```python
from build123d import *

# Parameters (mm, degrees)
SKETCH_W        = 57
SKETCH_H        = 42
PAD_DEPTH       = 2
SKETCH001_W     = 57
SKETCH001_H     = 42
SKETCH001_W_2   = 53
SKETCH001_H_2   = 38
PAD001_DEPTH    = 2
SKETCH002_R     = 4
PAD002_DEPTH    = 12
SKETCH003_R     = 3.25
POCKET_DEPTH    = 14
SKETCH004_R     = 1.5
PAD003_DEPTH    = 2
POCKET001_DEPTH = 3
SKETCH006_W     = 26.076656
SKETCH006_H     = 2.5
POCKET002_DEPTH = 1
POCKET003_DEPTH = 1
PAD004_DEPTH    = 1
PAD005_DEPTH    = 17
PAD006_DEPTH    = 1
SKETCH011_W     = 42
SKETCH011_H     = 14
PAD007_DEPTH    = 1
SKETCH012_R     = 3.5
POCKET004_DEPTH = 2
SKETCH013_W     = 18
SKETCH013_H     = 38
PAD008_DEPTH    = 1
SKETCH014_W     = 0.782134
SKETCH014_H     = 1
PAD009_DEPTH    = 2
POCKET005_DEPTH = 15
POCKET006_DEPTH = 15
POCKET007_DEPTH = 3
POCKET008_DEPTH = 3
POCKET009_DEPTH = 80
POCKET010_DEPTH = 80
POCKET011_DEPTH = 42
POCKET012_DEPTH = 42


with BuildPart() as part:
    # Sketch → Pad (new body)
    with BuildSketch(Plane.XY):
        Rectangle(SKETCH_W, SKETCH_H)
    extrude(amount=PAD_DEPTH)

    # Sketch001 (on Face6 of Pad) → Pad001 (join)
    with BuildSketch(Plane.XY.offset(2)):
        Rectangle(SKETCH001_W, SKETCH001_H)
        Rectangle(SKETCH001_W_2, SKETCH001_H_2, mode=Mode.SUBTRACT)
    extrude(amount=PAD001_DEPTH)

    # Sketch002 (on Face4 of Pad001) → Pad002 (join)
    with BuildSketch(Plane(origin=(0, 0, 0), x_dir=(1, 0, 0), z_dir=(0, 0, -1))):
        with Locations((-12, 0)):
            Circle(SKETCH002_R)
    pad002 = extrude(amount=PAD002_DEPTH)

    # Sketch003 (on Face12 of Pad002) → Pocket (cut)
    with BuildSketch(Plane(origin=(0, 0, -12), x_dir=(1, 0, 0), z_dir=(0, 0, -1))):
        with Locations((-12, 0)):
            Circle(SKETCH003_R)
    pocket = extrude(amount=-POCKET_DEPTH, mode=Mode.SUBTRACT)

    # Mirrored: Pad002 across Sketch002 V_Axis
    add(pad002.mirror(Plane(origin=(0, 0, 0), x_dir=(0, 0, -1), z_dir=(1, 0, 0))))

    # Mirrored001: Pocket across Sketch003 V_Axis
    add(pocket.mirror(Plane(origin=(0, 0, -12), x_dir=(0, 0, -1), z_dir=(1, 0, 0))), mode=Mode.SUBTRACT)

    # Sketch004 (on Face21 of Mirrored001) → Pad003 (join)
    with BuildSketch(Plane.XY.offset(2)):
        with Locations((0, 12.5)):
            Circle(SKETCH004_R)
    pad003 = extrude(amount=PAD003_DEPTH)

    # Mirrored002: Pad003 across Sketch004 H_Axis
    add(pad003.mirror(Plane(origin=(0, 0, 2), x_dir=(0, 0, 1), z_dir=(0, 1, 0))))

    # Sketch005 (on Face21 of Mirrored002) → Pocket001 (cut)
    with BuildSketch(Plane.XY.offset(4)):
        with BuildLine():
            ThreePointArc((14.048565, -2.52307), (15.249949, -0.018175), (14.076656, 2.5))
            Line((14.076656, 2.5), (28.5, 2.5))
            Line((28.5, 2.5), (28.5, -21))
            Line((28.5, -21), (14.048565, -2.52307))
        make_face()
    extrude(amount=-POCKET001_DEPTH, mode=Mode.SUBTRACT)

    # Sketch006 (on Face17 of Pocket001) → Pocket002 (cut)
    with BuildSketch(Plane.XY.offset(2)):
        with Locations((1.038328, 1.25)):
            Rectangle(SKETCH006_W, SKETCH006_H)
    extrude(amount=-POCKET002_DEPTH, mode=Mode.SUBTRACT)

    # Sketch007 (on Face13 of Pocket002) → Pocket003 (cut)
    with BuildSketch(Plane.XY.offset(4)):
        Polygon((28.5, 21), (28.5, 20), (-27.5, 20), (-27.5, -20), (28.5, -20), (28.5, -21), (-28.5, -21), (-28.5, 21), align=None)
    extrude(amount=-POCKET003_DEPTH, mode=Mode.SUBTRACT)

    # Sketch008 (on Face3 of Pocket003) → Pad004 (join)
    with BuildSketch(Plane.YZ.offset(28.5)):
        Polygon((-19, 1), (-19, 15), (-20, 15), (-20, 4), (-20, 3), (-21, 3), (-21, 0), (21, 0), (21, 3), (20, 3), (20, 15), (19, 15), (19, 1), align=None)
    extrude(amount=PAD004_DEPTH)

    # Sketch009 (on Face10 of Pad004) → Pad005 (join)
    with BuildSketch(Plane.YZ.offset(29.5)):
        Polygon((-19, 15), (-20, 15), (-20, 14), (-21, 14), (-21, 0), (21, 0), (21, 14), (20, 14), (20, 15), (19, 15), (19, 1), (-19, 1), align=None)
    extrude(amount=PAD005_DEPTH)

    # Sketch010 (on Face20 of Pad005) → Pad006 (join)
    with BuildSketch(Plane.YZ.offset(46.5)):
        Polygon((-20, 15), (20, 15), (20, 14), (21, 14), (21, 0), (-21, 0), (-21, 14), (-20, 14), align=None)
    extrude(amount=PAD006_DEPTH)

    # Sketch011 (on Face34 of Pad006) → Pad007 (join)
    with BuildSketch(Plane.YZ.offset(47.5)):
        with Locations((0, 7)):
            Rectangle(SKETCH011_W, SKETCH011_H)
    extrude(amount=PAD007_DEPTH)

    # Sketch012 (on Face51 of Pad007) → Pocket004 (cut)
    with BuildSketch(Plane.YZ.offset(48.5)):
        with Locations((0, 8.5)):
            Circle(SKETCH012_R)
    extrude(amount=-POCKET004_DEPTH, mode=Mode.SUBTRACT)

    # Sketch013 (on Face77 of Pocket004) → Pad008 (join)
    with BuildSketch(Plane.XY.offset(1)):
        with Locations((37.5, 0)):
            Rectangle(SKETCH013_W, SKETCH013_H)
    extrude(amount=PAD008_DEPTH)

    # Sketch014 (on Face40 of Pad008) → Pad009 (join)
    with BuildSketch(Plane.XY.offset(1)):
        with Locations((28.108933, -20.5)):
            Rectangle(SKETCH014_W, SKETCH014_H)
    extrude(amount=PAD009_DEPTH)

    # Sketch015 (on Face50 of Pad009) → Pocket005 (cut)
    with BuildSketch(Plane.XY.offset(14)):
        with BuildLine():
            ThreePointArc((47.018921, -21), (48.067334, -20.554064), (48.5, -19.500105))
            Line((48.5, -19.500105), (48.5, -21))
            Line((48.5, -21), (47.018921, -21))
        make_face()
    extrude(amount=-POCKET005_DEPTH, mode=Mode.SUBTRACT)

    # Sketch016 (on Face51 of Pocket005) → Pocket006 (cut)
    with BuildSketch(Plane.XY.offset(14)):
        with BuildLine():
            ThreePointArc((48.5, 19.5), (48.060658, 20.560658), (47, 21))
            Line((47, 21), (48.5, 21))
            Line((48.5, 21), (48.5, 19.5))
        make_face()
    extrude(amount=-POCKET006_DEPTH, mode=Mode.SUBTRACT)

    # Sketch017 (on Face13 of Pocket006) → Pocket007 (cut)
    with BuildSketch(Plane.XY.offset(3)):
        with BuildLine():
            ThreePointArc((-27, 21), (-28.060664, 20.560656), (-28.5, 19.499989))
            Line((-28.5, 21), (-28.5, 19.499989))
            Line((-27, 21), (-28.5, 21))
        make_face()
    extrude(amount=-POCKET007_DEPTH, mode=Mode.SUBTRACT)

    # Sketch018 (on Face13 of Pocket007) → Pocket008 (cut)
    with BuildSketch(Plane.XY.offset(3)):
        with BuildLine():
            ThreePointArc((-28.5, -19.466143), (-28.035422, -20.547385), (-26.949118, -21))
            Line((-28.5, -21), (-26.949118, -21))
            Line((-28.5, -19.466143), (-28.5, -21))
        make_face()
    extrude(amount=-POCKET008_DEPTH, mode=Mode.SUBTRACT)

    # Sketch019 (on Face60 of Pocket008) → Pocket009 (cut)
    with BuildSketch(Plane.YZ.offset(48.5)):
        with BuildLine():
            Line((-21.000105, 1.5), (-21.000105, 0))
            Line((-21.000105, 0), (-19.500105, 0))
            ThreePointArc((-21.000105, 1.5), (-20.560765, 0.43934), (-19.500105, 0))
        make_face()
    extrude(amount=-POCKET009_DEPTH, mode=Mode.SUBTRACT)

    # Sketch020 (on Face36 of Pocket009) → Pocket010 (cut)
    with BuildSketch(Plane.YZ.offset(48.5)):
        with BuildLine():
            Line((19.5, 0), (21, 0))
            Line((21, 0), (21, 1.5))
            ThreePointArc((19.5, 0), (20.56066, 0.43934), (21, 1.5))
        make_face()
    extrude(amount=-POCKET010_DEPTH, mode=Mode.SUBTRACT)

    # Sketch021 (on Face13 of Pocket010) → Pocket011 (cut)
    with BuildSketch(Plane(origin=(0, 21, 0), x_dir=(-1, 0, 0), z_dir=(0, 1, 0))):
        with BuildLine():
            Line((-48.5, 1.5), (-48.5, 0))
            Line((-47, 0), (-48.5, 0))
            ThreePointArc((-48.5, 1.5), (-48.06066, 0.43934), (-47, 0))
        make_face()
    extrude(amount=-POCKET011_DEPTH, mode=Mode.SUBTRACT)

    # Sketch022 (on Face4 of Pocket011) → Pocket012 (cut)
    with BuildSketch(Plane(origin=(0, 21, 0), x_dir=(-1, 0, 0), z_dir=(0, 1, 0))):
        with BuildLine():
            Line((28.5, 1.5), (28.5, 0))
            Line((28.5, 0), (27, 0))
            ThreePointArc((27, 0), (28.06066, 0.43934), (28.5, 1.5))
        make_face()
    extrude(amount=-POCKET012_DEPTH, mode=Mode.SUBTRACT)


solid = part.part
```
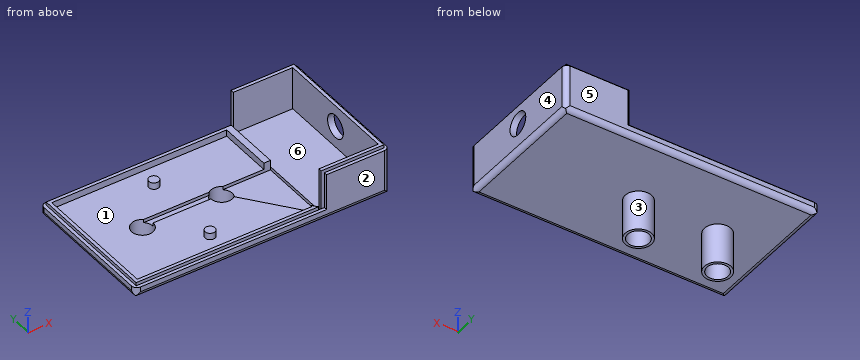
Verification items for the finished model (mm, model axes). Face numbers are marked on the shaded views. A direction names the side the tool comes from. Give positions to 0.01 mm unless a question says otherwise; leave off trailing zeros. Loops run counter-clockwise (first coordinate to the right, second up) from the corner with the lowest first, then second, coordinate; pieces in that order, holes last.
1. Go/stop test with flat-tipped pins: pin 1 Ø3 at (x, y) = (32, -10) entering from -Z; pin 2 Ø1.5 at (x, y) = (0.5, -12.5) entering from +Z; pin 3 Ø2 at (y, z) = (4.5, -7.5) entering from -X; pin 4 Ø6 at (x, y) = (12, 0) entering from -Z. Record where each tip stops, or that it passes through.
2. Set-up check for the marked faces 1, 2 and 3: record each of +Z, -Z, +X, -X, +Y, -Y from which the full face is reachable in a straight line by a thin tool's end or side.
3. Thickness scan on line 1 (X direction, y = 0, z = -9); line 2 (Y direction, x = -12, z = -2.5); line 3 (Z direction, x = 47, y = 0). Record the ranges inside material, lowest first.
4. Mould release check, pull along X, two halves, no side actions. Record for the marked faces 4, 5 and 6: released by +X, released by -X, zero draft, split by the parting line, or undercut.
5. Section check D-D, the plane z = -2.5. Enter the section's corners in (x, y).
6. Section check A-A, the plane z = 8.5. Enter the section's corners in (x, y), then the cut area to 3 significant figures.
7. Section check B-B, the plane x = 12. Enter the section's corners in (y, z).
8. Section check C-C, the plane y = 12.5. Enter the section's corners in (x, z), then the cut area to 3 significant figures.
Geometry says:
1. pin 1: stops at z = 0
1. pin 2: stops at z = 4
1. pin 3: stops at x = -13.94
1. pin 4: passes through
2. face 1: +Z
2. face 2: +Z, -Z, +X, -X, -Y
2. face 3: -Z
3. line 1: x = -16 to -15.25, -8.75 to -8, 8 to 8.75, 15.25 to 16
3. line 2: y = -4 to -3.25, 3.25 to 4
3. line 3: z = 0 to 5, 12 to 15
4. face 4: released by +X
4. face 5: zero draft
4. face 6: undercut
5. outline: circle Ø8 at (-12, 0); circle Ø8 at (12, 0); hole circle Ø6.5 at (-12, 0); hole circle Ø6.5 at (12, 0)
6. outline: (28.5, -20) - (29.5, -20) - (29.5, -21) - (47.02, -21) arc R1.5 ccw to (48.5, -19.5) - (48.5, -3.5) - (46.5, -3.5) - (46.5, -19) - (28.5, -19) - close; (28.5, 19) - (46.5, 19) - (46.5, 3.5) - (48.5, 3.5) - (48.5, 19.5) arc R1.5 ccw to (47, 21) - (29.5, 21) - (29.5, 20) - (28.5, 20) - close
6. area: 139 mm2
7. outline: (-21, 1.48) arc R1.5 ccw to (-19.5, 0) - (-4, 0) - (-4, -12) - (-3.25, -12) - (-3.25, 2) - (-19, 2) - (-19, 4) - (-20, 4) - (-20, 3) - (-21, 3) - close; (3.25, -12) - (4, -12) - (4, 0) - (19.5, 0) arc R1.5 ccw to (21, 1.5) - (21, 3) - (20, 3) - (20, 4) - (19, 4) - (19, 2) - (3.25, 2) - close
8. outline: (-28.5, 1.5) arc R1.5 ccw to (-27, 0) - (47, 0) arc R1.5 ccw to (48.5, 1.5) - (48.5, 14) - (47.5, 14) - (47.5, 15) - (46.5, 15) - (46.5, 2) - (28.5, 2) - (28.5, 4) - (26.5, 4) - (26.5, 2) - (1.5, 2) - (1.5, 4) - (-1.5, 4) - (-1.5, 2) - (-26.5, 2) - (-26.5, 4) - (-27.5, 4) - (-27.5, 3) - (-28.5, 3) - close
8. area: 191 mm2
